```python
from build123d import *

# Parameters (mm, degrees)
BOSS_EXTRUDE1_DEPTH   = 1.5875
BOSS_EXTRUDE3_DEPTH   = 25.4
FILLET2_R             = 0.508
F_4_CLEARANCE_HOLE1_D = 3.4544
CUT_EXTRUDE3_START    = -6.35
CUT_EXTRUDE3_DEPTH    = 4.7625
CHAMFER1_SIZE         = 2.54


with BuildPart() as part:
    # Sketch2 → Boss-Extrude1 (new body)
    with BuildSketch(Plane.XY):
        Polygon((-37.376757149, -111.329189904), (-34.092160805, -86.142458737), (-8.905429638, -89.427055082), (-12.190025983, -114.613786248), align=None)
    extrude(amount=BOSS_EXTRUDE1_DEPTH)

    # Sketch4 → Boss-Extrude3 (add)
    with BuildSketch(Plane(origin=(-11.61606456, -89.073561748, 0), x_dir=(0.9916035892333672, -0.12931481670521638, 0), z_dir=(0.12931481670521638, 0.9916035892333672, 0))):
        with BuildLine():
            Line((-22.666412757, -1.5875), (-12.484171192, -3.155171915))
            ThreePointArc((-12.484171192, -3.155171915), (-11.111427592, -3.611643646), (-9.966412757, -4.4958))
            Line((-9.966412757, -4.4958), (2.733587243, -1.5875))
            Line((2.733587243, -1.5875), (-22.666412757, -1.5875))
        make_face()
    extrude(amount=-BOSS_EXTRUDE3_DEPTH)

    # Fillet2
    fillet2_edges = [part.edges().sort_by_distance(p)[0] for p in [
        (-23.141093394, -100.378122493, 4.4958),
    ]]
    fillet(fillet2_edges, radius=FILLET2_R)

    # #4 Clearance Hole1 (through all)
    with Locations(Plane(origin=(0, 0, 0), x_dir=(-1, 0, 0), z_dir=(0, 0, -1))):
        with Locations((12.464345577, -92.164821934), (31.354393952, -89.701374676), (33.81784121, -108.591423051), (14.927792835, -111.054870309)):
            Hole(F_4_CLEARANCE_HOLE1_D / 2)

    # Sketch9 → Cut-Extrude3 (cut)
    with BuildSketch(Plane(origin=(0, 0, 0), x_dir=(-1, 0, 0), z_dir=(0, 0, -1)).offset(CUT_EXTRUDE3_START)):
        with BuildLine():
            Line((33.407266667, -105.443081655), (39.974131611, -104.586698171))
            Line((39.974131611, -104.586698171), (39.974131611, -116.083768321))
            Line((39.974131611, -116.083768321), (31.712540611, -117.000176181))
            Line((31.712540611, -117.000176181), (30.669499814, -109.001997594))
            ThreePointArc((30.669499814, -109.001997594), (31.301307616, -106.655529544), (33.407266667, -105.443081655))
        make_face()
        with BuildLine():
            Line((27.163011759, -82.113770632), (35.383316986, -80.880777852))
            Line((35.383316986, -80.880777852), (38.331833439, -91.993332588))
            Line((38.331833439, -91.993332588), (31.764968495, -92.849716072))
            ThreePointArc((31.764968495, -92.849716072), (29.418500445, -92.21790827), (28.206052556, -90.111949219))
            Line((28.206052556, -90.111949219), (27.163011759, -82.113770632))
        make_face()
        with BuildLine():
            Line((12.87492012, -95.31316333), (6.308055176, -96.169546814))
            Line((6.308055176, -96.169546814), (6.308055176, -84.672476664))
            Line((6.308055176, -84.672476664), (14.569646176, -83.756068805))
            Line((14.569646176, -83.756068805), (15.612686973, -91.754247391))
            ThreePointArc((15.612686973, -91.754247391), (14.980879171, -94.100715441), (12.87492012, -95.31316333))
        make_face()
        with BuildLine():
            Line((19.119175028, -118.642474353), (10.898869802, -119.875467134))
            Line((10.898869802, -119.875467134), (7.950353349, -108.762912398))
            Line((7.950353349, -108.762912398), (14.517218292, -107.906528913))
            ThreePointArc((14.517218292, -107.906528913), (16.863686342, -108.538336715), (18.076134231, -110.644295766))
            Line((18.076134231, -110.644295766), (19.119175028, -118.642474353))
        make_face()
    extrude(amount=CUT_EXTRUDE3_DEPTH, mode=Mode.SUBTRACT)

    # Chamfer1
    chamfer1_edges = [part.edges().sort_by_distance(p)[0] for p in [
        (-37.376757149, -111.329189904, 0.79375),
        (-34.092160805, -86.142458737, 0.79375),
        (-8.905429638, -89.427055082, 0.79375),
        (-12.190025983, -114.613786248, 0.79375),
    ]]
    chamfer(chamfer1_edges, length=CHAMFER1_SIZE)


solid = part.part
```
Input: part model. Units: mm. Frame: model coordinates. A direction names the side the tool comes from. Round coordinates to 2 decimals unless told otherwise and drop trailing zeros. Order: outer loops, then holes, each group sorted by start corner. A loop starts at its lowest first (then second) coordinate and runs counter-clockwise, first axis right, second up. Notation, with made-up numbers: (81.25, 82) - (92.25, 82) arc R25 cw to (92.25, 103) - close; hole circle Ø7 at (11, 11). An arc over 180 degrees is marked (long way). One line per question, with ' | ' between items. Start each with the question number.
1) Ray query, probe 1 along Y at (x, z) = (-16.25, 0.2); probe 2 along Z at (x, y) = (-32, -108.75); probe 3 along Y at (x, z) = (-19.5, 1.5). Return the intervals inside material, ascending.
2) Cut plane A-A, the plane x = -29.25. Return the cut outline in (y, z).
3) Set-up query: faces 5 (the flat face through (-18.28, -112.2, 2.32)), 6 (the cylindrical face through (-16.84, -108.52, 2.16)), 7 (the flat face through (-30.878, -110.598, 2.083)). Return all of +Z, -Z, +X, -X, +Y, -Y with unobstructed straight access to the full face (end or side cutting, diameter ignored); none if empty.
4) Pull-direction query (Y, two-part tool) for faces 1 (the cylindrical face through (-31.28, -106.683, 1.975)), 2 (the cylindrical face through (-33.021, -110.124, 0.805)), 3 (the cylindrical face through (-29.45, -92.24, 1.97)), 4 (the flat face through (-35.9, -110.3, 0.8)); classes: +Y half, -Y half, draft (parallel to the pull), parting line (faces both ways), or undercut.
5) Cut plane B-B, the plane z = 1.05. Return the cut outline in (x, y), then the cut area to 3 significant figures.
6) Contact query for flat-ended pins moving along their axis: P1, Ø1.5, axis at y = -95.5, z = 0.5, coming from the +X side; P2, Ø1.5, axis at y = -104.5, z = 1, coming from the +X side; P3, Ø7, axis at x = -16.5, y = -112.5, coming from the +Z side; P4, Ø3, axis at x = -33.82, y = -108.59, coming from the -Z side. Output: stop coordinate, or through.
7) Cut plane D-D, the plane z = 3.6. Return the cut outline in (x, y), then the cut area to 3 significant figures.
8) Cut plane C-C, the plane y = -91. Give the number of separate pieces and of enclosed holes in the cut face, then the cut area to 3 significant figures.
Worked out:
1) probe 1: y = -114.08 to -112.17, -109.94 to -88.47 | probe 2: z = 0 to 1.59 | probe 3: y = -113.66 to -88.05
2) outline: (-112.39, 0) - (-86.77, 0) - (-86.77, 1.59) - (-92.08, 1.59) - (-92.08, 2.44) - (-112.39, 2.85) - close
3) face 5: +Z, +X, -Y | face 6: +Z, -Y | face 7: +Z, -X
4) face 1: undercut | face 2: undercut | face 3: +Y half | face 4: -Y half
5) outline: (-37.05, -108.81) - (-34.86, -111.66) - (-14.71, -114.29) - (-11.86, -112.1) - (-9.23, -91.95) - (-11.42, -89.1) - (-31.57, -86.47) - (-34.42, -88.66) - close; hole circle Ø3.45 at (-33.82, -108.59); hole circle Ø3.45 at (-31.35, -89.7); hole circle Ø3.45 at (-14.93, -111.05); hole circle Ø3.45 at (-12.46, -92.16) | area: 595 mm^2
6) P1: stops at x = -9.6 | P2: stops at x = -10.77 | P3: stops at z = 3.43 | P4: passes through
7) outline: (-25.94, -112.82) - (-20.9, -113.48) - (-17.62, -88.29) - (-22.66, -87.63) - close | area: 129 mm^2
8) separate pieces: 3 | enclosed holes: 0 | area: 55.9 mm^2
